Source: CAD feature listing. Evaluate the final solid. Frame: model axes, mm. Coordinates: 2 decimals unless noted, no trailing zeros. Order: outer loops, then holes, each group sorted by start corner. A loop starts at its lowest first (then second) coordinate and runs counter-clockwise, first axis right, second up.
Item 1: Section C-C on y = -61. Return the cut outline in (x, z), then the cut area to 3 significant figures.
Item 2: Section A-A on x = 3. Return the cut outline in (y, z).
Item 3: Section B-B on z = 80. Return the cut outline in (x, y), then the cut area to 3 significant figures.
Item 4: Section D-D on z = 45.6. Return the cut outline in (x, y), then the cut area to 3 significant figures.
Item 5: Contact query for flat-ended pins moving along their axis: P1, Ø2, axis at x = 3, z = 45.6, coming from the +Y side; P2, Ø2, axis at y = -39.5, z = 52, coming from the -X side; P3, Ø2, axis at x = 5, z = 12, coming from the -Y side; P4, Ø2.5, axis at x = 3, z = 80, coming from the -Y side. Output: stop coordinate, or through.
Item 6: Ray query, line 1 (Z direction, x = 3, y = -15.25); line 2 (X direction, y = -86, z = 70); line 3 (Z direction, x = 3, y = -6). Return the intervals inside material, ascending.
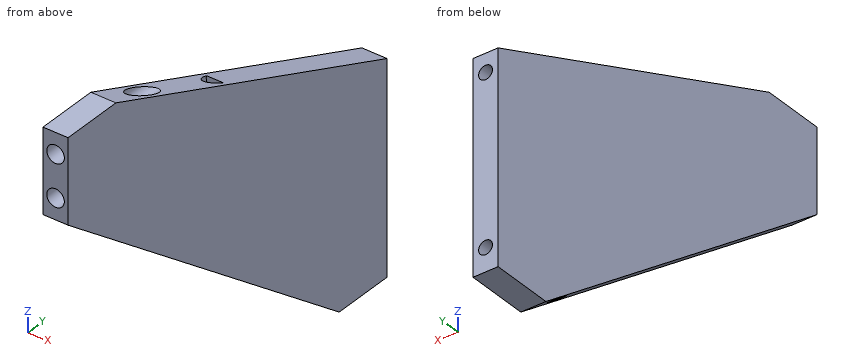
from build123d import *

# Parameters (mm, degrees)
F1_DEPTH = 6
F2_R     = 2.1
F3_DEPTH = 50
F4_R     = 1.65
F5_DEPTH = 30


with BuildPart() as f1:
    # F0 (on Right) → F1 (new body)
    with BuildSketch(Plane.YZ):
        Polygon((-15, 0), (0, 0), (0, 50), (-85, 85), (-100, 85), (-100, 65), align=None)
    extrude(amount=F1_DEPTH)

    # F2 (on face) → F3 (cut)
    with BuildSketch(Plane.XZ.offset(100)):
        with Locations((3, 70)):
            Circle(F2_R)
        with Locations((3, 80)):
            Circle(F2_R)
    extrude(amount=-F3_DEPTH, mode=Mode.SUBTRACT)

    # F4 (on face) → F5 (cut)
    with BuildSketch(Plane(origin=(0, 0, 0), x_dir=(-1, 0, 0), z_dir=(0, 1, 0))):
        with Locations((-3, 45.6)):
            Circle(F4_R)
        with Locations((-3, 5.6)):
            Circle(F4_R)
    extrude(amount=-F5_DEPTH, mode=Mode.SUBTRACT)


solid = f1.part
Answer list:
1. outline: (0, 35.18) - (6, 35.18) - (6, 75.12) - (0, 75.12) - close; hole circle Ø4.2 at (3, 70)
1. area: 226 mm2
2. outline: (-100, 65) - (-24.48, 7.25) - (0, 7.25) - (0, 43.95) - (-30, 43.95) - (-30, 47.25) - (0, 47.25) - (0, 50) - (-50, 70.59) - (-50, 67.9) - (-100, 67.9) - close; (-100, 72.1) - (-53.67, 72.1) - (-67.76, 77.9) - (-100, 77.9) - close; (-100, 82.1) - (-77.96, 82.1) - (-85, 85) - (-100, 85) - close; (-20.17, 3.95) - (-15, 0) - (0, 0) - (0, 3.95) - close
3. outline: (0, -100) - (0.9, -100) - (0.9, -72.86) - (0, -72.86) - close; (5.1, -100) - (6, -100) - (6, -72.86) - (5.1, -72.86) - close
3. area: 48.9 mm2
4. outline: (0, -74.63) - (6, -74.63) - (6, 0) - (4.65, 0) - (4.65, -30) - (1.35, -30) - (1.35, 0) - (0, 0) - close
4. area: 349 mm2
5. P1: stops at y = -30
5. P2: stops at x = 0
5. P3: stops at y = -32
5. P4: passes through
6. line 1: z = 0.19 to 3.95, 7.25 to 43.95, 47.25 to 56.28
6. line 2: x = 0 to 0.9, 5.1 to 6
6. line 3: z = 0 to 3.95, 7.25 to 43.95, 47.25 to 52.47
